from build123d import *

# Parameters (mm, degrees)
EXTRUDE_2_DEPTH      = 3
CUT_EXTRUDE_1_DEPTH  = 0.6
SKETCH_6_W           = 18
SKETCH_6_H           = 26
CUT_EXTRUDE_4_DEPTH  = 3.4
FILLET_1_R           = 1
CUT_EXTRUDE_6_DEPTH  = 3.4
FILLET_2_R           = 1
SKETCH_22_R          = 1.7
CUT_EXTRUDE_18_DEPTH = 4
SKETCH_23_R          = 3
CUT_EXTRUDE_19_DEPTH = 1


with BuildPart() as part:
    # 草图1 → 凸台-拉伸2 (new body)
    with BuildSketch(Plane.XY):
        with BuildLine():
            ThreePointArc((-4.008613189, 3.630478791), (-4.334307099, 3.328571786), (-4.497154053, 2.91540689))
            ThreePointArc((-4.497154053, 2.91540689), (-4.847622487, 1.898244021), (-5.534413817, 1.070134068))
            Line((-5.534413817, 1.070134068), (-8.898384051, -1.752572115))
            ThreePointArc((-8.898384051, -1.752572115), (-9.80068645, -2.273516648), (-10.82674688, -2.454438786))
            Line((-10.82674688, -2.454438786), (-51.498806412, -2.454438786))
            ThreePointArc((-51.498806412, -2.454438786), (-52.524866842, -2.273516648), (-53.427169241, -1.752572115))
            Line((-53.427169241, -1.752572115), (-56.791139475, 1.070134068))
            ThreePointArc((-56.791139475, 1.070134068), (-57.477930804, 1.898244021), (-57.828399238, 2.91540689))
            ThreePointArc((-57.828399238, 2.91540689), (-57.991246193, 3.328571786), (-58.316940102, 3.630478791))
            Line((-58.316940102, 3.630478791), (-65.723943689, 7.906914306))
            Line((-65.723943689, 7.906914306), (-65.723943689, 16.984208123))
            Line((-65.723943689, 16.984208123), (-58.316940102, 21.260643637))
            ThreePointArc((-58.316940102, 21.260643637), (-57.991246193, 21.562550642), (-57.828399238, 21.975715539))
            ThreePointArc((-57.828399238, 21.975715539), (-57.477930804, 22.992878408), (-56.791139475, 23.820988361))
            Line((-56.791139475, 23.820988361), (-53.427169241, 26.643694544))
            ThreePointArc((-53.427169241, 26.643694544), (-52.524866842, 27.164639077), (-51.498806412, 27.345561214))
            Line((-51.498806412, 27.345561214), (-10.82674688, 27.345561214))
            ThreePointArc((-10.82674688, 27.345561214), (-9.80068645, 27.164639077), (-8.898384051, 26.643694544))
            Line((-8.898384051, 26.643694544), (-5.534413817, 23.820988361))
            ThreePointArc((-5.534413817, 23.820988361), (-4.847622487, 22.992878408), (-4.497154053, 21.975715539))
            ThreePointArc((-4.497154053, 21.975715539), (-4.334307099, 21.562550642), (-4.008613189, 21.260643637))
            Line((-4.008613189, 21.260643637), (3.398390397, 16.984208123))
            Line((3.398390397, 16.984208123), (3.398390397, 7.906914306))
            Line((3.398390397, 7.906914306), (-4.008613189, 3.630478791))
        make_face()
        with BuildLine():
            ThreePointArc((-51.498806412, 26.345561214), (-52.182846698, 26.224946456), (-52.784381631, 25.8776501))
            Line((-52.784381631, 25.8776501), (-56.148351865, 23.054943918))
            ThreePointArc((-56.148351865, 23.054943918), (-56.67539222, 22.368091555), (-56.862776646, 21.522855031))
            Line((-56.862776646, 21.522855031), (-56.862776646, 3.368267397))
            ThreePointArc((-56.862776646, 3.368267397), (-56.67539222, 2.523030874), (-56.148351865, 1.836178511))
            Line((-56.148351865, 1.836178511), (-52.784381631, -0.986527672))
            ThreePointArc((-52.784381631, -0.986527672), (-52.182846698, -1.333824027), (-51.498806412, -1.454438786))
            Line((-51.498806412, -1.454438786), (-10.82674688, -1.454438786))
            ThreePointArc((-10.82674688, -1.454438786), (-10.142706593, -1.333824027), (-9.541171661, -0.986527672))
            Line((-9.541171661, -0.986527672), (-6.177201426, 1.836178511))
            ThreePointArc((-6.177201426, 1.836178511), (-5.650161072, 2.523030874), (-5.462776646, 3.368267397))
            Line((-5.462776646, 3.368267397), (-5.462776646, 21.522855031))
            ThreePointArc((-5.462776646, 21.522855031), (-5.650161072, 22.368091555), (-6.177201426, 23.054943918))
            Line((-6.177201426, 23.054943918), (-9.541171661, 25.8776501))
            ThreePointArc((-9.541171661, 25.8776501), (-10.142706593, 26.224946456), (-10.82674688, 26.345561214))
            Line((-10.82674688, 26.345561214), (-51.498806412, 26.345561214))
        make_face(mode=Mode.SUBTRACT)
        with BuildLine():
            Line((-10.82674688, 26.345561214), (-51.498806412, 26.345561214))
            ThreePointArc((-51.498806412, 26.345561214), (-52.182846698, 26.224946456), (-52.784381631, 25.8776501))
            Line((-52.784381631, 25.8776501), (-56.148351865, 23.054943918))
            ThreePointArc((-56.148351865, 23.054943918), (-56.67539222, 22.368091555), (-56.862776646, 21.522855031))
            Line((-56.862776646, 21.522855031), (-56.862776646, 3.368267397))
            ThreePointArc((-56.862776646, 3.368267397), (-56.67539222, 2.523030874), (-56.148351865, 1.836178511))
            Line((-56.148351865, 1.836178511), (-52.784381631, -0.986527672))
            ThreePointArc((-52.784381631, -0.986527672), (-52.182846698, -1.333824027), (-51.498806412, -1.454438786))
            Line((-51.498806412, -1.454438786), (-10.82674688, -1.454438786))
            ThreePointArc((-10.82674688, -1.454438786), (-10.142706593, -1.333824027), (-9.541171661, -0.986527672))
            Line((-9.541171661, -0.986527672), (-6.177201426, 1.836178511))
            ThreePointArc((-6.177201426, 1.836178511), (-5.650161072, 2.523030874), (-5.462776646, 3.368267397))
            Line((-5.462776646, 3.368267397), (-5.462776646, 21.522855031))
            ThreePointArc((-5.462776646, 21.522855031), (-5.650161072, 22.368091555), (-6.177201426, 23.054943918))
            Line((-6.177201426, 23.054943918), (-9.541171661, 25.8776501))
            ThreePointArc((-9.541171661, 25.8776501), (-10.142706593, 26.224946456), (-10.82674688, 26.345561214))
        make_face()
        with BuildLine():
            ThreePointArc((-53.78228524, 2.445561214), (-52.78228524, 3.445561214), (-53.78228524, 4.445561214))
            ThreePointArc((-53.78228524, 4.445561214), (-54.78228524, 3.445561214), (-53.78228524, 2.445561214))
        make_face(mode=Mode.SUBTRACT)
        with BuildLine():
            ThreePointArc((-53.78228524, 20.445561214), (-52.78228524, 21.445561214), (-53.78228524, 22.445561214))
            ThreePointArc((-53.78228524, 22.445561214), (-54.78228524, 21.445561214), (-53.78228524, 20.445561214))
        make_face(mode=Mode.SUBTRACT)
        with BuildLine():
            ThreePointArc((-8.58228524, 2.445561214), (-7.58228524, 3.445561214), (-8.58228524, 4.445561214))
            ThreePointArc((-8.58228524, 4.445561214), (-9.58228524, 3.445561214), (-8.58228524, 2.445561214))
        make_face(mode=Mode.SUBTRACT)
        with BuildLine():
            ThreePointArc((-8.58228524, 20.445561214), (-7.58228524, 21.445561214), (-8.58228524, 22.445561214))
            ThreePointArc((-8.58228524, 22.445561214), (-9.58228524, 21.445561214), (-8.58228524, 20.445561214))
        make_face(mode=Mode.SUBTRACT)
    extrude(amount=EXTRUDE_2_DEPTH)

    # 草图4 → 切除-拉伸1 (cut)
    with BuildSketch(Plane.XY.offset(3)):
        with BuildLine():
            Line((-56.148351865, 1.836178511), (-52.784381631, -0.986527672))
            ThreePointArc((-52.784381631, -0.986527672), (-52.182846698, -1.333824027), (-51.498806412, -1.454438786))
            Line((-51.498806412, -1.454438786), (-10.82674688, -1.454438786))
            ThreePointArc((-10.82674688, -1.454438786), (-10.142706593, -1.333824027), (-9.541171661, -0.986527672))
            Line((-9.541171661, -0.986527672), (-6.177201426, 1.836178511))
            ThreePointArc((-6.177201426, 1.836178511), (-5.71934054, 2.388251813), (-5.485694918, 3.066360392))
            ThreePointArc((-5.485694918, 3.066360392), (-5.160001008, 3.892690185), (-4.508613189, 4.496504195))
            Line((-4.508613189, 4.496504195), (-4.508613189, 20.394618234))
            ThreePointArc((-4.508613189, 20.394618234), (-5.160001008, 20.998432243), (-5.485694918, 21.824762036))
            ThreePointArc((-5.485694918, 21.824762036), (-5.71934054, 22.502870615), (-6.177201426, 23.054943918))
            Line((-6.177201426, 23.054943918), (-9.541171661, 25.8776501))
            ThreePointArc((-9.541171661, 25.8776501), (-10.142706593, 26.224946456), (-10.82674688, 26.345561214))
            Line((-10.82674688, 26.345561214), (-51.498806412, 26.345561214))
            ThreePointArc((-51.498806412, 26.345561214), (-52.182846698, 26.224946456), (-52.784381631, 25.8776501))
            Line((-52.784381631, 25.8776501), (-56.148351865, 23.054943918))
            ThreePointArc((-56.148351865, 23.054943918), (-56.606212752, 22.502870615), (-56.839858374, 21.824762036))
            ThreePointArc((-56.839858374, 21.824762036), (-57.165552284, 20.998432243), (-57.816940102, 20.394618234))
            Line((-57.816940102, 20.394618234), (-57.816940102, 4.496504195))
            ThreePointArc((-57.816940102, 4.496504195), (-57.165552284, 3.892690185), (-56.839858374, 3.066360392))
            ThreePointArc((-56.839858374, 3.066360392), (-56.606212752, 2.388251813), (-56.148351865, 1.836178511))
        make_face()
    extrude(amount=-CUT_EXTRUDE_1_DEPTH, mode=Mode.SUBTRACT)

    # 草图6 → 切除-拉伸4 (cut, through all)
    with BuildSketch(Plane.XY.offset(2.4)):
        with Locations((-20.162776646, 12.445561214)):
            Rectangle(SKETCH_6_W, SKETCH_6_H)
        with Locations((-42.162776646, 12.445561214)):
            Rectangle(SKETCH_6_W, SKETCH_6_H)
    extrude(amount=-CUT_EXTRUDE_4_DEPTH, mode=Mode.SUBTRACT)

    # 圆角1
    fillet_1_edges = [part.edges().sort_by_distance(p)[0] for p in [
        (-29.162776646, -0.554438786, 1.2),
        (-29.162776646, 25.445561214, 1.2),
        (-33.162776646, 25.445561214, 1.2),
        (-33.162776646, -0.554438786, 1.2),
    ]]
    fillet(fillet_1_edges, radius=FILLET_1_R)

    # 草图10 → 切除-拉伸6 (cut, through all)
    with BuildSketch(Plane.XY.offset(2.4)):
        Polygon((-11.162776646, 7.249408791), (-11.162776646, 17.641713637), (-6.662776646, 15.043637426), (-6.662776646, 9.847485003), align=None)
        Polygon((-51.162776646, 7.249408791), (-51.162776646, 17.641713637), (-55.662776646, 15.043637426), (-55.662776646, 9.847485003), align=None)
    extrude(amount=-CUT_EXTRUDE_6_DEPTH, mode=Mode.SUBTRACT)

    # 圆角2
    fillet_2_edges = [part.edges().sort_by_distance(p)[0] for p in [
        (-11.162776646, 25.445561214, 1.2),
        (-11.162776646, -0.554438786, 1.2),
        (-51.162776646, -0.554438786, 1.2),
        (-51.162776646, 25.445561214, 1.2),
    ]]
    fillet(fillet_2_edges, radius=FILLET_2_R)

    # 草图22 → 切除-拉伸18 (cut, through all)
    with BuildSketch(Plane.XY.offset(3)):
        with Locations((-1.162776646, 12.445561214)):
            Circle(SKETCH_22_R)
        with Locations((-61.162776646, 12.445561214)):
            Circle(SKETCH_22_R)
    extrude(amount=-CUT_EXTRUDE_18_DEPTH, mode=Mode.SUBTRACT)

    # 草图23 → 切除-拉伸19 (cut)
    with BuildSketch(Plane(origin=(0, 0, 0), x_dir=(-1, 0, 0), z_dir=(0, 0, -1))):
        with Locations((53.78228524, 3.445561214)):
            Circle(SKETCH_23_R)
        with Locations((53.78228524, 21.445561214)):
            Circle(SKETCH_23_R)
        with Locations((8.58228524, 21.445561214)):
            Circle(SKETCH_23_R)
        with Locations((8.58228524, 3.445561214)):
            Circle(SKETCH_23_R)
    extrude(amount=-CUT_EXTRUDE_19_DEPTH, mode=Mode.SUBTRACT)


solid = part.part
Geometry: final body of the model. Coordinates: model frame, mm. A direction names the side the tool comes from. Round coordinates to 2 decimals unless told otherwise and drop trailing zeros. Loops run counter-clockwise (first coordinate to the right, second up) from the corner with the lowest first, then second, coordinate; pieces in that order, holes last. Notation, with made-up numbers: (39, 35) - (55, 35) arc R19 cw to (55, 64) - close; hole circle Ø7 at (-15, -36.5). An arc over 180 degrees is marked (long way). Write each question's results on one line, items separated by ' | '. Start each with the question number.
1) Line query: probe 1 along Y at (x, z) = (-48, 0.65); probe 2 along X at (y, z) = (22.75, 1.15); probe 3 along Y at (x, z) = (-14, 2.6). Output: solid intervals per line, ascending. Write a range as [from, to].
2) Access query for faces 1 (the face through (-7.7, 4.2, 1)), 2 (the face through (-20, -0.554, 1)), 3 (the face through (-57.47, 1.885, 1.479)). Directions: +Z, -Z, +X, -X, +Y, -Y. A direction counts if a zero-diameter tool reaches every point of the face in a straight line with its end or side. Return the directions, or none.
3) Cut plane A-A on x = -40.5. Return loops of the section in (y, z).
4) First-contact query: P1, Ø5, axis at x = -8.58, y = 3.45, coming from the +Z side; P2, Ø4, axis at x = -36.5, y = 4, coming from the +Z side; P3, Ø2.5, axis at x = -8.58, y = 21.45, coming from the -Z side; P4, Ø1.5, axis at x = -57.5, z = 2, coming from the -Y side. Flat tips, straight axial feed; report the tip coordinate or a pass-through.
5) Cut plane C-C on z = 0.45. Count the separate pieces of the cut face and the enclosed holes in it, then the cut area to 3 significant figures.
6) Cut plane B-B on y = 11.5. Return loops of the section in (x, z), then the cut area to 3 significant figures.
7) Mould query, pull axis Y, two halves, no side actions, for faces 4 (the face through (-52.54, 27.16, 1.48)), 5 (the face through (-31, -2.454, 1)), 6 (the face through (-8.94, 16.36, 1.22)). Classes: released by +Y, released by -Y, zero draft, split by the parting line, or undercut.
Verdict:
1) probe 1: y = [-2.45, -0.55], [25.45, 27.35] | probe 2: x = [-57.6, -51.16], [-33.16, -29.16], [-11.16, -4.73] | probe 3: y = [-2.45, -1.45], [26.35, 27.35]
2) face 1: -Z | face 2: +Z, -Z | face 3: +Z, -Z, -X, -Y
3) outline: (-2.45, 0) - (-0.55, 0) - (-0.55, 2.4) - (-1.45, 2.4) - (-1.45, 3) - (-2.45, 3) - close; (25.45, 0) - (27.35, 0) - (27.35, 3) - (26.35, 3) - (26.35, 2.4) - (25.45, 2.4) - close
4) P1: stops at z = 2.4 | P2: passes through | P3: stops at z = 1 | P4: stops at y = 1.04
5) separate pieces: 1 | enclosed holes: 4 | area: 625 mm2
6) outline: (-65.72, 0) - (-62.58, 0) - (-62.58, 3) - (-65.72, 3) - close; (-59.75, 0) - (-55.66, 0) - (-55.66, 2.4) - (-57.82, 2.4) - (-57.82, 3) - (-59.75, 3) - close; (-33.16, 0) - (-29.16, 0) - (-29.16, 2.4) - (-33.16, 2.4) - close; (-6.66, 0) - (-2.58, 0) - (-2.58, 3) - (-4.51, 3) - (-4.51, 2.4) - (-6.66, 2.4) - close; (0.25, 0) - (3.4, 0) - (3.4, 3) - (0.25, 3) - close | area: 50.4 mm2
7) face 4: released by +Y | face 5: released by -Y | face 6: undercut
